```python
from build123d import *

# Parameters (mm, degrees)
SKETCH1_W               = 55
SKETCH1_H               = 125
BOSS_EXTRUDE1_DEPTH     = 50
FILLET1_SIZE            = 15
CHAMFER1_SIZE           = 15
SHELL1_T                = -3
SKETCH11_W              = 10
SKETCH11_H              = 29
BOSS_EXTRUDE3_DEPTH     = 5
CUT_EXTRUDE2_DEPTH      = 133.876822659
CUT_EXTRUDE2_DEPTH_BACK = 133.876822659
SKETCH12_W              = 3
SKETCH12_H              = 25
SKETCH31_R              = 14.5
BOSS_EXTRUDE10_DEPTH    = 8
SKETCH32_R              = 13.5
CUT_EXTRUDE11_DEPTH     = 8
SKETCH33_R              = 9.5
CUT_EXTRUDE12_DEPTH     = 20
SKETCH34_R              = 2.5
CUT_EXTRUDE15_DEPTH     = 5
SKETCH39_W              = 15
SKETCH39_H              = 11
SKETCH39_W_2            = 25
CUT_EXTRUDE16_DEPTH     = 10
SKETCH41_R              = 6.25
SKETCH41_R_2            = 5.25
CUT_EXTRUDE17_DEPTH     = 10
SKETCH44_R              = 1.5
BOSS_EXTRUDE11_DEPTH    = 3
SKETCH45_R              = 1.5
BOSS_EXTRUDE12_DEPTH    = 3.5


with BuildPart() as part:
    # Sketch1 → Boss-Extrude1 (new body)
    with BuildSketch(Plane(origin=(0, 0, 0), x_dir=(1, 0, 0), z_dir=(0, 1, 0))):
        with Locations((27.5, -62.5)):
            Rectangle(SKETCH1_W, SKETCH1_H)
    extrude(amount=BOSS_EXTRUDE1_DEPTH)

    # Fillet1
    fillet1_edges = [part.edges().sort_by_distance(p)[0] for p in [
        (55, 0, 62.5),
    ]]
    chamfer(fillet1_edges, length=FILLET1_SIZE)

    # Chamfer1
    chamfer1_edges = [part.edges().sort_by_distance(p)[0] for p in [
        (0, 0, 62.5),
    ]]
    chamfer(chamfer1_edges, length=CHAMFER1_SIZE)

    # Shell1
    shell1_openings = [part.faces().sort_by_distance(p)[0] for p in [
        (27.5, 50, 62.5),
    ]]
    offset(amount=SHELL1_T, openings=shell1_openings, kind=Kind.INTERSECTION)

    # Sketch11 → Boss-Extrude3 (add)
    with BuildSketch(Plane(origin=(55, 0, 0), x_dir=(0, 0, -1), z_dir=(1, 0, 0))):
        with Locations((-102.5, 32.5)):
            Rectangle(SKETCH11_W, SKETCH11_H)
        with Locations((-22.5, 32.5)):
            Rectangle(SKETCH11_W, SKETCH11_H)
    extrude(amount=BOSS_EXTRUDE3_DEPTH)

    # Sketch12 → Cut-Extrude2 (cut, two sides: drawn at the far end of the back side and taken through both)
    with BuildSketch(Plane.XY.offset(107.5).offset(-CUT_EXTRUDE2_DEPTH_BACK)):
        with Locations((56.5, 32.5)):
            Rectangle(SKETCH12_W, SKETCH12_H)
    extrude(amount=CUT_EXTRUDE2_DEPTH + CUT_EXTRUDE2_DEPTH_BACK, mode=Mode.SUBTRACT)

    # Sketch31 → Boss-Extrude10 (add)
    with BuildSketch(Plane.XY.offset(125)):
        with Locations((19, 30)):
            Circle(SKETCH31_R)
    extrude(amount=BOSS_EXTRUDE10_DEPTH)

    # Sketch32 → Cut-Extrude11 (cut)
    with BuildSketch(Plane.XY.offset(133)):
        with Locations((19, 30)):
            Circle(SKETCH32_R)
    extrude(amount=-CUT_EXTRUDE11_DEPTH, mode=Mode.SUBTRACT)

    # Sketch33 → Cut-Extrude12 (cut)
    with BuildSketch(Plane.XY.offset(125)):
        with Locations((19, 30)):
            Circle(SKETCH33_R)
    extrude(amount=-CUT_EXTRUDE12_DEPTH, mode=Mode.SUBTRACT)

    # Sketch34 → Cut-Extrude15 (cut)
    with BuildSketch(Plane.XY.offset(125)):
        with Locations((45, 30)):
            Circle(SKETCH34_R)
    extrude(amount=-CUT_EXTRUDE15_DEPTH, mode=Mode.SUBTRACT)

    # Sketch39 → Cut-Extrude16 (cut)
    with BuildSketch(Plane.ZY):
        with Locations((47.5, 23.5)):
            Rectangle(SKETCH39_W, SKETCH39_H)
        with Locations((82.5, 23.5)):
            Rectangle(SKETCH39_W_2, SKETCH39_H)
    extrude(amount=-CUT_EXTRUDE16_DEPTH, mode=Mode.SUBTRACT)

    # Sketch41 → Cut-Extrude17 (cut)
    with BuildSketch(Plane.ZY):
        with Locations((62.5, 40)):
            Circle(SKETCH41_R)
        with Locations((27, 40)):
            Circle(SKETCH41_R_2)
    extrude(amount=-CUT_EXTRUDE17_DEPTH, mode=Mode.SUBTRACT)

    # Sketch44 → Boss-Extrude11 (add)
    with BuildSketch(Plane(origin=(3, 0, 0), x_dir=(0, 0, -1), z_dir=(1, 0, 0))):
        with Locations((-87, 46.5)):
            Circle(SKETCH44_R)
    extrude(amount=BOSS_EXTRUDE11_DEPTH)

    # Sketch45 → Boss-Extrude12 (add)
    with BuildSketch(Plane.ZY.offset(-52)):
        with Locations((38, 46.5)):
            Circle(SKETCH45_R)
    extrude(amount=BOSS_EXTRUDE12_DEPTH)


solid = part.part
```
The model under review builds one solid part; all positions refer to its coordinate system, in mm. A direction names the side the tool comes from. Coordinates: 2 decimals unless noted, no trailing zeros. Order: outer loops, then holes, each group sorted by start corner. A loop starts at its lowest first (then second) coordinate and runs counter-clockwise, first axis right, second up. Notation, with made-up numbers: (35.25, 34.5) -> (56.25, 34.5) arc R22 ccw to (56.25, 59.5) -> close; hole circle Ø9 at (28.25, -3.75). An arc over 180 degrees is marked (long way). Answer in a Markdown table with one row per item. Add a question column.
Item 1: Mouldability with a two-part tool opening along X and no side actions: class faces 1 (the flat face through (56, 45, 22)), 2 (the flat face through (1, 23, 40)), 3 (the flat face through (7, 8, 63)) as +X half, -X half, draft (parallel to the pull), parting line (faces both ways), or undercut.
Item 2: To check wall thickness, follow probe 1 along X at (y, z) = (42.5, 101); probe 2 along Z at (x, y) = (22.5, 5); probe 3 along X at (y, z) = (39, 85.5). State the ranges of each line that lie inside material, in increasing order.
Item 3: We need section D-D on z = 52. Write out the cut boundary in (x, y), plus the area to 3 significant figures.
Item 4: Clearance check with flat-ended pins moving along their axes: pin 1 (1.5 mm diameter, centred on x = 50, y = 8.5, fed in from -Z); pin 2 (0.9 mm diameter, centred on x = 56.5, z = 24, fed in from +Y); pin 3 (11 mm diameter, centred on y = 40, z = 62.5, fed in from +X); pin 4 (0.9 mm diameter, centred on x = 2, z = 48.5, fed in from -Y). State where each tip first meets the part, or that it passes through.
Item 5: We need section B-B on y = 8.5. Write out the cut boundary in (x, z), plus the area to 3 significant figures.
Item 6: Machinability: for faces 4 (the flat face through (1, 29, 47)), 5 (the flat face through (59, 32, 97.5)), 6 (the flat face through (48.5, 47, 38)), which of the approach directions +Z, -Z, +X, -X, +Y, -Y give a long, thin tool a straight path to every point of the face, cutting with its end or side? Answer none if there is none.
Item 7: We need section C-C on x = 45. Write out the cut boundary in (y, z), plus the area to 3 significant figures.
Item 8: We need section A-A on z = 87. Write out the cut boundary in (x, y).
Final values:
| question | item | result |
|---|---|---|
| 1 | face 1 | undercut |
| 1 | face 2 | draft |
| 1 | face 3 | -X half |
| 2 | probe 1 | x = 0 to 3, 52 to 55, 58 to 60 |
| 2 | probe 2 | z = 0 to 3, 122 to 125 |
| 2 | probe 3 | x = 0 to 3, 52 to 55 |
| 3 | outline | (0, 15) -> (15, 0) -> (40, 0) -> (55, 15) -> (55, 50) -> (52, 50) -> (52, 16.24) -> (38.76, 3) -> (16.24, 3) -> (3, 16.24) -> (3, 18) -> (0, 18) -> close; (0, 29) -> (3, 29) -> (3, 50) -> (0, 50) -> close |
| 3 | area | 364 mm2 |
| 4 | pin 1 | passes through |
| 4 | pin 2 | stops at y = 47 |
| 4 | pin 3 | stops at x = 55 |
| 4 | pin 4 | stops at y = 12.55 |
| 5 | outline | (6.5, 0) -> (48.5, 0) -> (48.5, 125) -> (6.5, 125) -> close; hole (10.74, 3) -> (44.26, 3) -> (44.26, 122) -> (10.74, 122) -> close |
| 5 | area | 1,260 mm2 |
| 6 | face 4 | -X |
| 6 | face 5 | +X, +Y, -Y |
| 6 | face 6 | +Y |
| 7 | outline | (5, 0) -> (50, 0) -> (50, 3) -> (9.24, 3) -> (9.24, 122) -> (27.5, 122) -> (27.5, 125) -> (5, 125) -> close; (32.5, 122) -> (50, 122) -> (50, 125) -> (32.5, 125) -> close |
| 7 | area | 760 mm2 |
| 8 | outline | (0, 15) -> (15, 0) -> (40, 0) -> (55, 15) -> (55, 50) -> (52, 50) -> (52, 16.24) -> (38.76, 3) -> (16.24, 3) -> (3, 16.24) -> (3, 18) -> (0, 18) -> close; (0, 29) -> (3, 29) -> (3, 45) -> (6, 45) -> (6, 48) -> (3, 48) -> (3, 50) -> (0, 50) -> close |
